Geometry: final body of the model. Coordinates: model frame, mm. Give positions to 0.01 mm unless a question says otherwise; leave off trailing zeros. Loops run counter-clockwise (first coordinate to the right, second up) from the corner with the lowest first, then second, coordinate; pieces in that order, holes last. Notation, with made-up numbers: (84.5, 60.5) -> (103.5, 60.5) arc R22 ccw to (103.5, 67.5) -> close; hole circle Ø7 at (-9.75, -2). An arc over 180 degrees is marked (long way). One line per question, with ' | ' between items. Start each with the question number.
Item 1: Pin query (flat end, axial travel): P1, Ø1.6, axis at x = -64, y = 1, coming from the +Z side; P2, Ø1.6, axis at y = 1, z = 63, coming from the +X side; P3, Ø1.5, axis at y = 4.5, z = -31.5, coming from the -X side; P4, Ø5.5, axis at x = 0, z = 67, coming from the -Y side. Return the tip coordinate at first contact, or that it passes through.
Item 2: Section A-A on z = 48.5. Return loops of the section in (x, y), then the cut area to 3 significant figures.
Item 3: Material intervals for line 1 along Z through (x, y) = (0, 0.45); line 2 along Z through (x, y) = (-67, 0.4), sorted ascending. Write a range as [from, to].
Item 4: Section C-C on y = 4. Return loops of the section in (x, z).
Item 5: Section D-D on z = -61.5. Return loops of the section in (x, y), then the cut area to 3 significant figures.
Item 6: Section B-B on x = -34.5. Return loops of the section in (y, z).
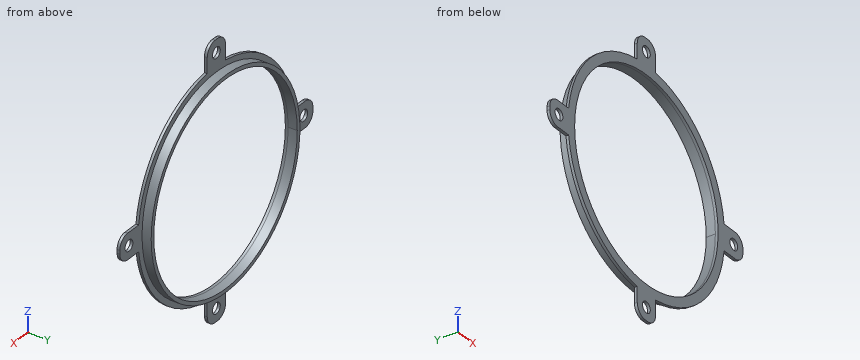
Autodesk Inventor part; units mm, degrees
ref_plane "YZ Plane" through (0, 0, 0) normal (1, 0, 0) x (0, 1, 0)
ref_plane "XZ Plane" through (0, 0, 0) normal (0, 1, 0) x (-1, 0, 0)
ref_plane "XY Plane" through (0, 0, 0) normal (0, 0, 1) x (1, 0, 0)
sketch "Sketch1" plane through (0, 0, 0) normal (0, 1, 0) x (-1, 0, 0)
  circle A0 centre (0, 0) radius 55
  circle A1 centre (0, 0) radius 60
  line L0 (0, 57.5) -> (7, 57.5)
  line L1 (7, 57.5) -> (-7, 57.5)
  line L2 (7, 57.5) -> (-7, 57.5)
  line L3 (-7, 57.5) -> (-7, 74)
  line L4 (-7, 74) -> (7, 74)
  line L5 (7, 74) -> (7, 57.5)
  line L6 (-74, 7) -> (-57.5, 7)
  line L7 (-74, -7) -> (-74, 7)
  line L8 (-57.5, -7) -> (-74, -7)
  line L9 (-57.5, 7) -> (-57.5, -7)
  line L10 (-7, -74) -> (-7, -57.5)
  line L11 (7, -74) -> (-7, -74)
  line L12 (7, -57.5) -> (7, -74)
  line L13 (-7, -57.5) -> (7, -57.5)
  line L14 (74, -7) -> (57.5, -7)
  line L15 (74, 7) -> (74, -7)
  line L16 (57.5, 7) -> (74, 7)
  line L17 (57.5, -7) -> (57.5, 7)
  point P0 (-7, 59.5903)
  point P1 (-59.5903, 7)
  point P2 (-59.5903, -7)
  point P3 (-7, -59.5903)
  point P4 (7, -59.5903)
  point P5 (59.5903, -7)
  point P6 (59.5903, 7)
  point P7 (7, 59.5903)
  dimension "d0" = 110
  dimension "d1" = 120
  dimension "d2" = 7
  dimension "d3" = 14
  dimension "d7" = 360
extrude "Extrusion1" add sketch "Sketch1" along normal blind 1.5
fillet "Fillet1" radius 6 8 edges at (74, 0.75, -7) (74, 0.75, 7) (7, 0.75, -74) (-7, 0.75, -74) (-74, 0.75, -7) (-74, 0.75, 7) (-7, 0.75, 74) (7, 0.75, 74)
sketch "Sketch2" plane through (0, 1.5, 0) normal (0, 1, 0) x (1, 0, 0)
  line L0 (-1, -74) -> (1, -74)
  line L1 (0, -74) -> (0, -67)
  line L2 (74, -1) -> (74, 1)
  line L3 (74, 0) -> (67, 0)
  line L4 (1, 74) -> (-1, 74)
  line L5 (0, 74) -> (0, 67)
  line L6 (-74, 1) -> (-74, -1)
  line L7 (-74, 0) -> (-67, 0)
  point P0 (0, 0)
  dimension "d12" = 7
  dimension "d13" = 7
  dimension "d14" = 7
  dimension "d15" = 7
hole "Hole1" at (0, 1.5, 67) at (-67, 1.5, 0) at (0, 1.5, -67) at (67, 1.5, 0) direction (0, -1, 0) diameter 6 end through all
sketch "Sketch3" plane through (0, 1.5, 0) normal (0, 1, 0) x (1, 0, 0)
  circle A0 centre (0, 0) radius 55
  circle A1 centre (0, 0) radius 55
  line L0 (-55, 0) -> (-57, 0)
  circle A2 centre (0, 0) radius 57
  dimension "d23" = 2
extrude "Extrusion2" add sketch "Sketch3" along normal blind 5
properties part number "Fan_Part2"
Result sheet:
1) P1: stops at z = 7 | P2: stops at x = 7 | P3: stops at x = -47.99 | P4: passes through
2) outline: (-35.32, 0) -> (-25.94, 0) -> (-25.94, 6.5) -> (-29.95, 6.5) -> (-29.95, 1.5) -> (-35.32, 1.5) -> close; (25.94, 0) -> (35.32, 0) -> (35.32, 1.5) -> (29.95, 1.5) -> (29.95, 6.5) -> (25.94, 6.5) -> close | area: 68.2 mm²
3) line 1: z = [-74, -70], [-64, -55], [55, 64], [70, 74] | line 2: z = [-7, -3], [3, 7]
4) outline: circle Ø114 at (0, 0); hole circle Ø110 at (0, 0)
5) outline: (-7, 0) -> (7, 0) -> (7, 1.5) -> (-7, 1.5) -> close | area: 21.0 mm²
6) outline: (0, -49.09) -> (1.5, -49.09) -> (1.5, -45.37) -> (6.5, -45.37) -> (6.5, -42.83) -> (0, -42.83) -> close; (0, 42.83) -> (6.5, 42.83) -> (6.5, 45.37) -> (1.5, 45.37) -> (1.5, 49.09) -> (0, 49.09) -> close
